The listing builds one solid part. Answer for the finished solid, in the listing's coordinates (mm). Coordinates: 2 decimals unless noted, no trailing zeros. Loops run counter-clockwise (first coordinate to the right, second up) from the corner with the lowest first, then second, coordinate; pieces in that order, holes last. Notation, with made-up numbers: (4.25, -39.75) - (59.25, -39.75) arc R19 cw to (59.25, -20.75) - close; hole circle Ø3 at (19.25, 62.5). An arc over 180 degrees is marked (long way). Put each result on its own line as item: value.
```python
from build123d import *

# Parameters (mm, degrees)
SKETCH1_R           = 2.6
SKETCH1_R_2         = 3
BOSS_EXTRUDE1_DEPTH = 12
FILLET1_R           = 5
FILLET2_R           = 6


with BuildPart() as part:
    # Sketch1 → Boss-Extrude1 (new body)
    with BuildSketch(Plane(origin=(0, 0, 0), x_dir=(1, 0, 0), z_dir=(0, 1, 0))):
        Polygon((180, 22), (155, 30), (35, 30), (15, 33), (0, 33), (-16, 12), (-16, 0), (0, 0), (155, 0), (180, 8), align=None)
        with Locations((-9, 6)):
            Circle(SKETCH1_R, mode=Mode.SUBTRACT)
        with Locations((148, 15)):
            Circle(SKETCH1_R_2, mode=Mode.SUBTRACT)
        with Locations((32, 15)):
            Circle(SKETCH1_R_2, mode=Mode.SUBTRACT)
        with Locations((175, 15)):
            Circle(SKETCH1_R, mode=Mode.SUBTRACT)
        with Locations((4, 25)):
            Circle(SKETCH1_R, mode=Mode.SUBTRACT)
    extrude(amount=BOSS_EXTRUDE1_DEPTH)

    # Fillet1
    fillet1_edges = [part.edges().sort_by_distance(p)[0] for p in [
        (-16, 6, 0),
    ]]
    fillet(fillet1_edges, radius=FILLET1_R)

    # Fillet2
    fillet2_edges = [part.edges().sort_by_distance(p)[0] for p in [
        (180, 6, -22),
        (180, 6, -8),
        (155, 6, 0),
    ]]
    fillet(fillet2_edges, radius=FILLET2_R)


solid = part.part
```
1) For a pull along Z with two mould halves and no side action, classify faces 1 (the face through (96, 6, -30)), 2 (the face through (70, 6, 0)), 3 (the face through (150.77, 5.92, -13.85)) as pulls with the +Z half, pulls with the -Z half, needs draft (parallel to the pull), parting line crosses it, or undercut.
Found:
face 1: pulls with the -Z half
face 2: pulls with the +Z half
face 3: undercut
2) Straight lines are drawn through the part: L1, parallel to X at y = 6, z = -13; L2, parallel to X at y = 2.75, z = -17; L3, parallel to Z at x = 32, y = 4. For each, find the intervals that lie inside material, in ascending order. Write a range as [from, to].
Found:
L1: x = [-15.24, 29.76], [34.24, 145.76], [150.24, 173.34], [176.66, 180]
L2: x = [-12.19, 29.76], [34.24, 145.76], [150.24, 173.34], [176.66, 180]
L3: z = [-30.45, -18], [-12, 0]
3) The part is cut by section C-C (x = 32). Give the vertices of the cut face in (y, z).
Found:
outline: (0, -30.45) - (12, -30.45) - (12, -18) - (0, -18) - close; (0, -12) - (12, -12) - (12, 0) - (0, 0) - close
4) The part is cut by section A-A (x = 4). Give the vertices of the cut face in (y, z), and give its area (3 significant figures).
Found:
outline: (0, -33) - (12, -33) - (12, -27.6) - (0, -27.6) - close; (0, -22.4) - (12, -22.4) - (12, 0) - (0, 0) - close
area: 334 mm^2
5) The part is cut by section D-D (z = -15). Give the vertices of the cut face in (x, y), and give its area (3 significant figures).
Found:
outline: (-13.71, 0) - (29, 0) - (29, 12) - (-13.71, 12) - close; (35, 0) - (145, 0) - (145, 12) - (35, 12) - close; (151, 0) - (172.4, 0) - (172.4, 12) - (151, 12) - close; (177.6, 0) - (180, 0) - (180, 12) - (177.6, 12) - close
area: 2,120 mm^2
6) Each of these flat-tipped pins is pushed along its axis until it touches: pin 1 (8.5 mm diameter, centred on x = 175, z = -15, fed in from -Y); pin 2 (4 mm diameter, centred on x = 66, y = 4, fed in from -Z). Where does it stop, or does it pass through?
Found:
pin 1: stops at y = 0
pin 2: stops at z = -30
7) The part is cut by section B-B (y = 10). Give the vertices of the cut face in (x, z).
Found:
outline: (-16, -12) - (0, -33) - (15, -33) - (35, -30) - (155, -30) - (175.83, -23.33) arc R6 ccw to (180, -17.62) - (180, -12.38) arc R6 ccw to (175.83, -6.67) - (155.89, -0.29) arc R6 ccw to (154.06, 0) - (-11, 0) arc R5 ccw to (-16, -5) - close; hole circle Ø5.2 at (-9, -6); hole circle Ø5.2 at (4, -25); hole circle Ø6 at (32, -15); hole circle Ø6 at (148, -15); hole circle Ø5.2 at (175, -15)
